The figure shows three views and two pictorial views of one solid part (mm, origin at its lowest corner). Answer the questions. A direction names the side the tool comes from. Coordinates: 2 decimals unless noted, no trailing zeros. Loops run counter-clockwise (first coordinate to the right, second up) from the corner with the lowest first, then second, coordinate; pieces in that order, holes last. Notation, with made-up numbers: M 11,25.25 L 70,25.25 A15 cw 70,50.25 Z; hole C 34,17 d4. An arc over 180 degrees is marked long. Write each question's results on one line, items separated by ' | '.
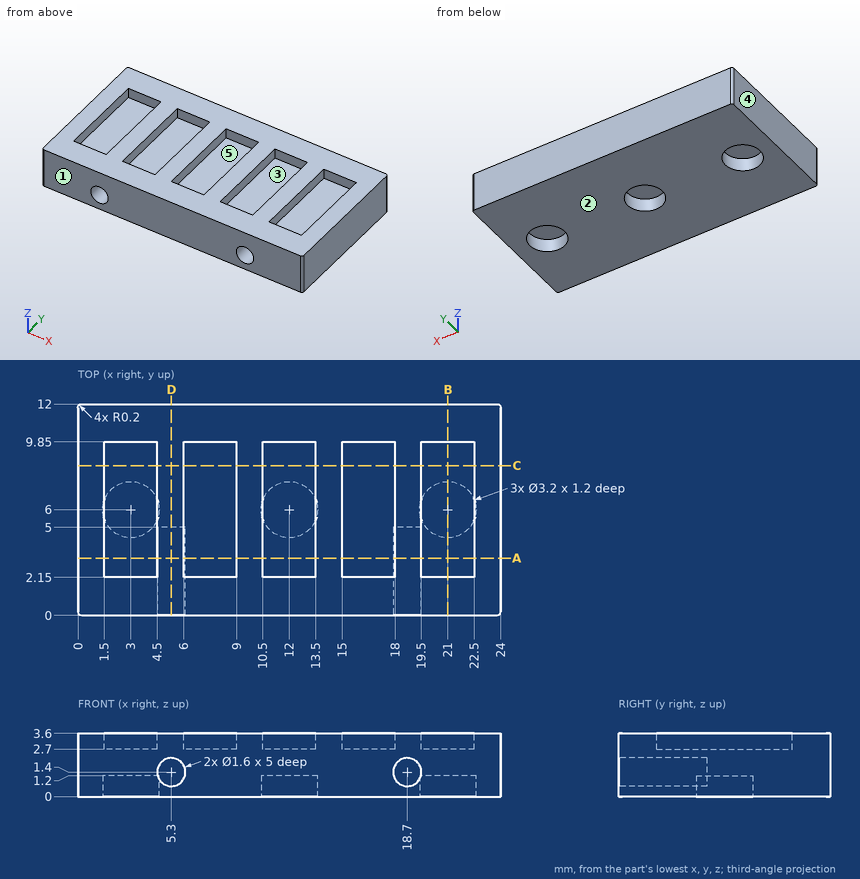
1) Find section B-B, the plane x = 21. Give the vertices of the cut face in (y, z), and give its area (3 significant figures).
Check result:
outline: M 0,0 L 4.4,0 L 4.4,1.2 L 7.6,1.2 L 7.6,0 L 12,0 L 12,3.6 L 9.85,3.6 L 9.85,2.7 L 2.15,2.7 L 2.15,3.6 L 0,3.6 Z | area: 32.4 mm^2
2) Find section A-A, the plane y = 3.25. Give the vertices of the cut face in (x, z).
Check result:
outline: M 0,0 L 24,0 L 24,3.6 L 22.5,3.6 L 22.5,2.7 L 19.5,2.7 L 19.5,3.6 L 18,3.6 L 18,2.7 L 15,2.7 L 15,3.6 L 13.5,3.6 L 13.5,2.7 L 10.5,2.7 L 10.5,3.6 L 9,3.6 L 9,2.7 L 6,2.7 L 6,3.6 L 4.5,3.6 L 4.5,2.7 L 1.5,2.7 L 1.5,3.6 L 0,3.6 Z; hole C 5.3,1.4 d1.6; hole C 18.7,1.4 d1.6
3) Straight lines are drawn through the part: probe 1 along X at (y, z) = (6, 0.6); probe 2 along X at (y, z) = (6, 2.85); probe 3 along Y at (x, z) = (3, 0.6). For each, find the intervals that lie inside material, in ascending order. Write a range as [from, to].
Check result:
probe 1: [0, 1.4], [4.6, 10.4], [13.6, 19.4], [22.6, 24] | probe 2: [0, 1.5], [4.5, 6], [9, 10.5], [13.5, 15], [18, 19.5], [22.5, 24] | probe 3: [0, 4.4], [7.6, 12]
4) For a pull along Y with two mould halves and no side action, classify the marked faces 1, 2 and 3 as released by +Y, released by -Y, zero draft, split by the parting line, or undercut.
Check result:
face 1: released by -Y | face 2: zero draft | face 3: undercut
5) Find section D-D, the plane x = 5.3. Give the vertices of the cut face in (y, z), and give its area (3 significant figures).
Check result:
outline: M 0,0 L 12,0 L 12,3.6 L 0,3.6 L 0,2.2 L 5,2.2 L 5,0.6 L 0,0.6 Z | area: 35.2 mm^2
6) Which of the six approach directions +Z, -Z, +X, -X, +Y, -Y give full straight-line access (tool end or side, diameter ignored) to the marked faces 4 and 5?
Check result:
face 4: +Z, -Z, -X, +Y, -Y | face 5: +Z
7) Given pin 1 Ø0.9 at (x, y) = (21.5, 5.5) entering from +Z, flat-ended and moving along its own axis, determine where the tip first touches the part or whether it passes through.
Check result:
pin 1: z = 2.7
8) Find section C-C, the plane y = 8.5. Give the vertices of the cut face in (x, z), and give its area (3 significant figures).
Check result:
outline: M 0,0 L 24,0 L 24,3.6 L 22.5,3.6 L 22.5,2.7 L 19.5,2.7 L 19.5,3.6 L 18,3.6 L 18,2.7 L 15,2.7 L 15,3.6 L 13.5,3.6 L 13.5,2.7 L 10.5,2.7 L 10.5,3.6 L 9,3.6 L 9,2.7 L 6,2.7 L 6,3.6 L 4.5,3.6 L 4.5,2.7 L 1.5,2.7 L 1.5,3.6 L 0,3.6 Z | area: 72.9 mm^2
